CAD build for the part. Positions are in the model's coordinates, mm. Face numbers are marked on the shaded views. A direction names the side the tool comes from. Give positions to 0.01 mm unless a question says otherwise; leave off trailing zeros. Write each loop counter-clockwise with the first axis right and the second up, starting at its lowest first coordinate (ties: lowest second). Pieces come first, ordered by that corner, then holes. Notation, with made-up numbers: M 21.5,-39.5 L 73.5,-39.5 A24 cw 73.5,-19.5 Z; hole C -31,48 d3. An arc over 180 degrees is marked long. One line per question, with ' | ' between items. Start each with the question number.
1. Which spindle directions (+Z, -Z, +X, -X, +Y, -Y) get a long thin tool onto all of the face, cutting with end or side? Do the marked faces 4, 5, 6 and 7. Say none if no direction does.
2. Pull direction Y, two halves, no side cores. Call the marked faces 1, 2 and 3: released by +Y, released by -Y, zero draft, split by the parting line, or undercut.
3. Cut at A-A, the plane y = 0. Write the cut outline in (x, z), then the cut area to 3 significant figures.
4. Flat gauge pins, fed straight in: pin 1 (5 mm diameter, centred on y = 5.5, z = -6.5, fed in from +X); pin 2 (1.5 mm diameter, centred on x = 5.5, z = -10, fed in from -Y); pin 3 (3.5 mm diameter, centred on x = -0.5, z = -7.5, fed in from -Y); pin 4 (1 mm diameter, centred on x = 5.5, y = -9, fed in from -Z). Where does each tip first touch, or does it go through?
5. Cut at B-B, the plane x = 0. Write the cut outline in (y, z), then the cut area to 3 significant figures.
6. Wall check: L1, parallel to X at y = 0, z = -5.7; L2, parallel to X at y = 0, z = -8.75; L3, parallel to X at y = -4.75, z = -0.25. Give the ranges that are in metal, low to high.
7. Cut at C-C, the plane z = -3.5. Write the cut outline in (x, y), then the cut area to 3 significant figures.
8. Cut at D-D, the plane x = 4.75. Write the cut outline in (y, z), then the cut area to 3 significant figures.
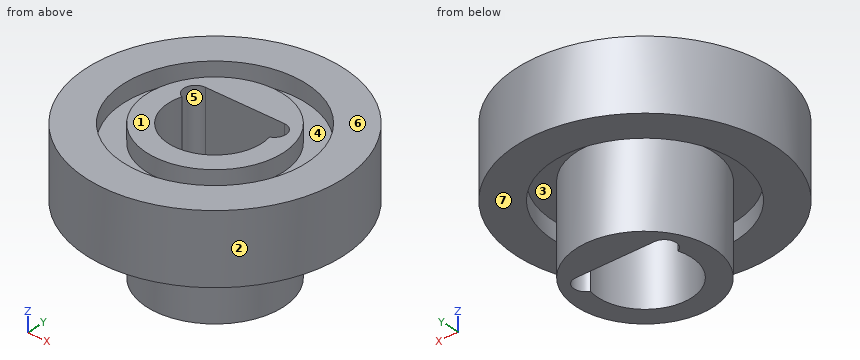
Autodesk Inventor part; units mm, degrees
ref_plane "YZ Plane" through (0, 0, 0) normal (1, 0, 0) x (0, 1, 0)
ref_plane "XZ Plane" through (0, 0, 0) normal (0, 1, 0) x (-1, 0, 0)
ref_plane "XY Plane" through (0, 0, 0) normal (0, 0, 1) x (1, 0, 0)
sketch "Esquisse1" plane through (0, 0, 0) normal (1, 0, 0) x (0, 1, 0)
  line L0 (0, 21.0755) -> (0, -24.2543)
  line L1 (7.85, -1.5) -> (7.85, 0)
  line L2 (7.85, 0) -> (11, 0)
  line L3 (11, 0) -> (11, -6)
  line L4 (11, -6) -> (7.85, -6)
  line L5 (7.85, -6) -> (7.85, -4.5)
  line L6 (7.85, -4.5) -> (5.85, -4.5)
  line L7 (5.85, -4.5) -> (5.85, -12)
  line L8 (5.85, -12) -> (2.5, -12)
  line L9 (7.85, -1.5) -> (5.85, -1.5)
  line L10 (5.85, -1.5) -> (5.85, 0)
  line L11 (5.85, 0) -> (2.5, 0)
  line L12 (2.5, 0) -> (2.5, -12)
  line L13 (6.85, -1.5) -> (6.85, -4.5) construction
  line L14 (6.85, -3) -> (11, -3) construction
  point P0 (0, 0)
  point P1 (7.85, -5.25)
  dimension "d0" = 11.7
  dimension "d1" = 5
  dimension "d2" = 12
  dimension "d3" = 6
  dimension "d4" = 22
  dimension "d5" = 2
  dimension "d6" = 3
revolve "Révolution1" add sketch "Esquisse1" angle 360 about axis through (0, 0, 21.0755) along (0, 0, -1)
sketch "Esquisse2" plane through (0, 0, 0) normal (0, 0, 1) x (1, 0, 0)
  arc A0 (-2.6458, 3) -> (-3.8519, 1.0783) centre (0, 0) ccw construction
  line L0 (-3.4641, 2) -> (3.4641, 2) construction
  line L1 (-3.4641, 1) -> (3.4641, 1) construction
  line L2 (3.4641, 3) -> (-3.4641, 3)
  arc A1 (-3.4641, 3) -> (-3.8519, 1.0783) centre (-3.4641, 2) ccw
  arc A2 (3.4641, 1) -> (3.8519, 1.0783) centre (3.4641, 2) ccw construction
  arc A3 (-3.8519, 1.0783) -> (-3.4641, 1) centre (-3.4641, 2) ccw construction
  arc A4 (3.8519, 1.0783) -> (3.4641, 3) centre (3.4641, 2) ccw
  arc A5 (2.6458, 3) -> (-2.6458, 3) centre (0, 0) ccw construction
  arc A6 (-3.8519, 1.0783) -> (3.8519, 1.0783) centre (0, 0) ccw
  arc A7 (3.8519, 1.0783) -> (2.6458, 3) centre (0, 0) ccw construction
  point P0 (0, 2)
  dimension "d9" = 1
  dimension "d11" = 3
  dimension "d12" = 4
extrude "Extrusion1" cut sketch "Esquisse2" against normal through all
properties part number "engrenage_simplifie_v3"
Here are the results:
1) face 4: +Z | face 5: +Z, -Z | face 6: +Z, +X, -X, +Y, -Y | face 7: -Z
2) face 1: zero draft | face 2: split by the parting line | face 3: undercut
3) outline: M -11,-6 L -7.85,-6 L -7.85,-4.5 L -5.85,-4.5 L -5.85,-12 L -4,-12 L -4,0 L -5.85,0 L -5.85,-1.5 L -7.85,-1.5 L -7.85,0 L -11,0 Z; M 4,-12 L 5.85,-12 L 5.85,-4.5 L 7.85,-4.5 L 7.85,-6 L 11,-6 L 11,0 L 7.85,0 L 7.85,-1.5 L 5.85,-1.5 L 5.85,0 L 4,0 Z | area: 94.2 mm^2
4) pin 1: x = 10.57 | pin 2: y = -3.41 | pin 3: y = -11 | pin 4: z = -6
5) outline: M -11,-6 L -7.85,-6 L -7.85,-4.5 L -5.85,-4.5 L -5.85,-12 L -4,-12 L -4,0 L -5.85,0 L -5.85,-1.5 L -7.85,-1.5 L -7.85,0 L -11,0 Z; M 3,-12 L 5.85,-12 L 5.85,-4.5 L 7.85,-4.5 L 7.85,-6 L 11,-6 L 11,0 L 7.85,0 L 7.85,-1.5 L 5.85,-1.5 L 5.85,0 L 3,0 Z | area: 106 mm^2
6) L1: -11 to -7.85, -5.85 to -4, 4 to 5.85, 7.85 to 11 | L2: -5.85 to -4, 4 to 5.85 | L3: -9.92 to -6.25, -3.41 to 3.41, 6.25 to 9.92
7) outline: C 0,0 d22; hole M -3.85,1.08 A4 ccw long 3.85,1.08 A1 ccw 3.46,3 L -3.46,3 A1 ccw Z | area: 330 mm^2
8) outline: M -9.92,-6 L -6.25,-6 L -6.25,-4.5 L -3.41,-4.5 L -3.41,-12 L 3.41,-12 L 3.41,-4.5 L 6.25,-4.5 L 6.25,-6 L 9.92,-6 L 9.92,0 L 6.25,0 L 6.25,-1.5 L 3.41,-1.5 L 3.41,0 L -3.41,0 L -3.41,-1.5 L -6.25,-1.5 L -6.25,0 L -9.92,0 Z | area: 143 mm^2
